from build123d import *

# Parameters (mm, degrees)
SKETCH_1_R          = 9.5
EXTRUDE_1_DEPTH     = 10
SKETCH_2_R          = 8.5
SKETCH_2_R_2        = 9.5
CUT_EXTRUDE_1_DEPTH = 5
SKETCH_3_R          = 3.25
SKETCH_3_R_2        = 2
EXTRUDE_2_DEPTH     = 5
SKETCH_4_W          = 16
SKETCH_4_H          = 2
CUT_EXTRUDE_2_DEPTH = 6
EXTRUDE_3_DEPTH     = 29.5
SKETCH_8_W          = 40
SKETCH_8_H          = 59
CUT_EXTRUDE_4_DEPTH = 8
SKETCH_9_R          = 9.5
CUT_EXTRUDE_5_DEPTH = 70
SKETCH_10_R         = 3.25
SKETCH_10_R_2       = 2
EXTRUDE_4_DEPTH     = 6


with BuildPart() as part:
    # Эскиз1 → Бобышка-Вытянуть1 (new body)
    with BuildSketch(Plane(origin=(0, 0, 0), x_dir=(1, 0, 0), z_dir=(0, 1, 0))):
        with BuildLine():
            Line((-20, 18), (20, 18))
            ThreePointArc((20, 18), (27.071067812, 15.071067812), (30, 8))
            Line((30, 8), (30, -2))
            ThreePointArc((30, -2), (27.071067812, -9.071067812), (20, -12))
            Line((20, -12), (-20, -12))
            ThreePointArc((-20, -12), (-27.071067812, -9.071067812), (-30, -2))
            Line((-30, -2), (-30, 8))
            ThreePointArc((-30, 8), (-27.071067812, 15.071067812), (-20, 18))
        make_face()
        with Locations(Location((-10, 0, 0), (0, 0, 270))):
            Circle(SKETCH_1_R, mode=Mode.SUBTRACT)
        with Locations(Location((10, 0, 0), (0, 0, 90))):
            Circle(SKETCH_1_R, mode=Mode.SUBTRACT)
    extrude_1 = extrude(amount=EXTRUDE_1_DEPTH)

    # Эскиз2 → Вырез-Вытянуть1 (cut)
    with BuildSketch(Plane(origin=(0, 10, 0), x_dir=(1, 0, 0), z_dir=(0, 1, 0))):
        with Locations((-20, -2)):
            Circle(SKETCH_2_R)
        with Locations((-20, 8)):
            Circle(SKETCH_2_R)
        with Locations(Location((-10, 0, 0), (0, 0, 270))):
            Circle(SKETCH_2_R_2)
        with BuildLine():
            Line((20, 16.5), (-20, 16.5))
            ThreePointArc((-20, 16.5), (-14.492370575, 14.474258113), (-11.609926002, 9.362592497))
            ThreePointArc((-11.609926002, 9.362592497), (-3.878084328, 7.26444413), (-0.5, 0))
            ThreePointArc((-0.5, 0), (-5.086783087, -8.13082404), (-14.417957802, -8.410210988))
            ThreePointArc((-14.417957802, -8.410210988), (-17.01979811, -9.960426917), (-20, -10.5))
            Line((-20, -10.5), (20, -10.5))
            ThreePointArc((20, -10.5), (17.01979811, -9.960426917), (14.417957802, -8.410210988))
            ThreePointArc((14.417957802, -8.410210988), (0.616398255, -1.48257151), (11.609926002, 9.362592497))
            ThreePointArc((11.609926002, 9.362592497), (14.492370575, 14.474258113), (20, 16.5))
        make_face()
        with Locations((-20, -2)):
            Circle(SKETCH_2_R)
        with Locations((-20, 8)):
            Circle(SKETCH_2_R)
        with Locations(Location((-10, 0, 0), (0, 0, 270))):
            Circle(SKETCH_2_R_2)
        with Locations((-20, -2)):
            Circle(SKETCH_2_R)
        with Locations((-20, 8)):
            Circle(SKETCH_2_R)
        with Locations(Location((-10, 0, 0), (0, 0, 270))):
            Circle(SKETCH_2_R_2)
        with BuildLine():
            ThreePointArc((-26.873863542, 3), (-28.08324935, 5.371106707), (-28.5, 8))
            Line((-28.5, 8), (-28.5, -2))
            ThreePointArc((-28.5, -2), (-28.08324935, 0.628893293), (-26.873863542, 3))
        make_face()
        with Locations((20, -2)):
            Circle(SKETCH_2_R)
        with Locations((20, 8)):
            Circle(SKETCH_2_R)
        with Locations(Location((10, 0, 0), (0, 0, 90))):
            Circle(SKETCH_2_R_2)
        with Locations((20, -2)):
            Circle(SKETCH_2_R)
        with Locations((20, 8)):
            Circle(SKETCH_2_R)
        with Locations(Location((10, 0, 0), (0, 0, 90))):
            Circle(SKETCH_2_R_2)
        with Locations((20, -2)):
            Circle(SKETCH_2_R)
        with Locations((20, 8)):
            Circle(SKETCH_2_R)
        with Locations(Location((10, 0, 0), (0, 0, 90))):
            Circle(SKETCH_2_R_2)
        with BuildLine():
            Line((28.5, -2), (28.5, 8))
            ThreePointArc((28.5, 8), (28.08324935, 5.371106707), (26.873863542, 3))
            ThreePointArc((26.873863542, 3), (28.08324935, 0.628893293), (28.5, -2))
        make_face()
    cut_extrude_1 = extrude(amount=-CUT_EXTRUDE_1_DEPTH, mode=Mode.SUBTRACT)

    # Эскиз3 → Бобышка-Вытянуть2 (add)
    with BuildSketch(Plane(origin=(0, 5, 0), x_dir=(1, 0, 0), z_dir=(0, 1, 0))):
        with Locations(Location((-23.5, 3, 0), (0, 0, 270))):
            Circle(SKETCH_3_R)
        with Locations(Location((-23.5, 3, 0), (0, 0, 270))):
            Circle(SKETCH_3_R_2, mode=Mode.SUBTRACT)
        with Locations(Location((23.5, 3, 0), (0, 0, 90))):
            Circle(SKETCH_3_R)
        with Locations(Location((23.5, 3, 0), (0, 0, 90))):
            Circle(SKETCH_3_R_2, mode=Mode.SUBTRACT)
    extrude_2 = extrude(amount=EXTRUDE_2_DEPTH)

    # Эскиз4 → Вырез-Вытянуть2 (cut, through all)
    with BuildSketch(Plane(origin=(0, 5, 0), x_dir=(1, 0, 0), z_dir=(0, 1, 0))):
        with Locations((0, 14)):
            Rectangle(SKETCH_4_W, SKETCH_4_H)
    cut_extrude_2 = extrude(amount=-CUT_EXTRUDE_2_DEPTH, mode=Mode.SUBTRACT)

    # Эскиз5 → Бобышка-Вытянуть3 (add)
    with BuildSketch(Plane.XZ):
        with BuildLine():
            Line((30, -8), (30, 2))
            ThreePointArc((30, 2), (27.071067812, 9.071067812), (20, 12))
            Line((20, 12), (-20, 12))
            ThreePointArc((-20, 12), (-27.071067812, 9.071067812), (-30, 2))
            Line((-30, 2), (-30, -8))
            ThreePointArc((-30, -8), (-27.071067812, -15.071067812), (-20, -18))
            Line((-20, -18), (20, -18))
            ThreePointArc((20, -18), (27.071067812, -15.071067812), (30, -8))
        make_face()
    extrude_3 = extrude(amount=EXTRUDE_3_DEPTH)

    # Зеркальное отражение5: Бобышка-Вытянуть1, Вырез-Вытянуть1, Бобышка-Вытянуть2, Вырез-Вытянуть2, Бобышка-Вытянуть3 across plane
    add(extrude_1.mirror(Plane(origin=(0, -29.5, 0), x_dir=(0, 0, 1), z_dir=(0, -1, 0))))
    add(cut_extrude_1.mirror(Plane(origin=(0, -29.5, 0), x_dir=(0, 0, 1), z_dir=(0, -1, 0))), mode=Mode.SUBTRACT)
    add(extrude_2.mirror(Plane(origin=(0, -29.5, 0), x_dir=(0, 0, 1), z_dir=(0, -1, 0))))
    add(cut_extrude_2.mirror(Plane(origin=(0, -29.5, 0), x_dir=(0, 0, 1), z_dir=(0, -1, 0))), mode=Mode.SUBTRACT)
    add(extrude_3.mirror(Plane(origin=(0, -29.5, 0), x_dir=(0, 0, 1), z_dir=(0, -1, 0))))

    # Эскиз8 → Вырез-Вытянуть4 (cut)
    with BuildSketch(Plane(origin=(0, 0, -18), x_dir=(-1, 0, 0), z_dir=(0, 0, -1))):
        with Locations((0, -29.5)):
            Rectangle(SKETCH_8_W, SKETCH_8_H)
    extrude(amount=-CUT_EXTRUDE_4_DEPTH, mode=Mode.SUBTRACT)

    # Эскиз9 → Вырез-Вытянуть5 (cut, through all)
    with BuildSketch(Plane(origin=(0, -59, 0), x_dir=(-1, 0, 0), z_dir=(0, -1, 0))):
        with Locations(Location((10, 0, 0), (0, 0, 270))):
            Circle(SKETCH_9_R)
        with Locations(Location((-10, 0, 0), (0, 0, 270))):
            Circle(SKETCH_9_R)
    extrude(amount=-CUT_EXTRUDE_5_DEPTH, mode=Mode.SUBTRACT)

    # Эскиз10 → Бобышка-Вытянуть4 (add)
    with BuildSketch(Plane(origin=(0, 0, -10), x_dir=(-1, 0, 0), z_dir=(0, 0, -1))):
        with Locations((-13.5, -52.5)):
            Circle(SKETCH_10_R)
        with Locations((-13.5, -52.5)):
            Circle(SKETCH_10_R_2, mode=Mode.SUBTRACT)
        with Locations(Location((13.5, -52.5, 0), (0, 0, 180))):
            Circle(SKETCH_10_R)
        with Locations(Location((13.5, -52.5, 0), (0, 0, 180))):
            Circle(SKETCH_10_R_2, mode=Mode.SUBTRACT)
        with Locations((13.5, -6.5)):
            Circle(SKETCH_10_R)
        with Locations((13.5, -6.5)):
            Circle(SKETCH_10_R_2, mode=Mode.SUBTRACT)
        with Locations(Location((-13.5, -6.5, 0), (0, 0, 180))):
            Circle(SKETCH_10_R)
        with Locations(Location((-13.5, -6.5, 0), (0, 0, 180))):
            Circle(SKETCH_10_R_2, mode=Mode.SUBTRACT)
    extrude(amount=EXTRUDE_4_DEPTH)


solid = part.part
Verification items for the finished model (mm, model axes). A direction names the side the tool comes from. Give positions to 0.01 mm unless a question says otherwise; leave off trailing zeros. Order: outer loops, then holes, each group sorted by start corner. A loop starts at its lowest first (then second) coordinate and runs counter-clockwise, first axis right, second up. Notation, with made-up numbers: M 38.5,46 L 66.5,46 A28 ccw 66.5,78 Z; hole C -25,58.5 d11. An arc over 180 degrees is marked long. Use one line per item in the form item = value. Start each with the question number.
Q1. Section check D-D (y = -11). Enter the section's corners in (x, z).
Q2. Scan lines: line 1 along X through (y, z) = (-61.05, 0); line 2 along Z through (x, y) = (9.5, -63.5); line 3 along Y through (x, z) = (13.5, -13.85). Record each from-to range of solid material in increasing order. Write a range as [from, to].
Q3. Section check B-B (x = 2.5). Enter the section's corners in (y, z).
Q4. Section check C-C (z = 4.75). Enter the section's corners in (x, y), then the cut area to 3 significant figures.
Q5. Access from +Z, -Z, +X, -X, +Y, -Y to the whole of each face (thin tool, end or side, straight path). Record for faces 4 (the flat face through (0, -64, -6)), 5 (the cylindrical face through (26.08, 7.54, -13.94)), 6 (the cylindrical face through (-14.205, -49.327, -12.958)), 7 (the flat face through (-26, -69, -3)), 8 (the flat face through (30, -30, -3)).
Q6. Mould release check, pull along Z, two halves, no side actions. Record for faces 1 (the flat face through (11, -52, -16)), 2 (the flat face through (0, -67, -16.5)), 3 (the cylindrical face through (14.205, -55.673, -12.958)): +Z half, -Z half, draft (parallel to the pull), parting line (faces both ways), or undercut.
Q7. Section check A-A (y = -52.5). Enter the section's corners in (x, z).
Q8. Go/stop test with flat-tipped pins: pin 1 Ø3 at (x, z) = (24.5, -2.5) entering from -Y; pin 2 Ø2 at (x, y) = (-3, -26.5) entering from -Z; pin 3 Ø17 at (x, z) = (-10, 0) entering from -Y; pin 4 Ø3 at (x, z) = (-23.5, -3) entering from -Y. Record where each tip stops, or that it passes through.
Evaluation:
q1.outline = M -30,-8 A10 ccw -20,-18 L -20,-10 L 20,-10 L 20,-18 A10 ccw 30,-8 L 30,2 A10 ccw 20,12 L -20,12 A10 ccw -30,2 Z; hole C -10,0 d19; hole C 10,0 d19
q2.line_1 = [-30, -19.5], [-0.5, 0.5], [19.5, 30]
q2.line_2 = [-18, -9.49], [9.49, 12]
q2.line_3 = [-64, -59], [-55.75, -54.5], [-50.5, -49.25], [-9.75, -8.5], [-4.5, -3.25], [0, 5]
q3.outline = M -69,-18 L -59,-18 L -59,-15 L -64,-15 L -64,-16.5 L -69,-16.5 Z; M -69,10.5 L -64,10.5 L -64,5.83 L 5,5.83 L 5,10.5 L 10,10.5 L 10,12 L -69,12 Z; M -64,-13 L -59,-13 L -59,-10 L 0,-10 L 0,-13 L 5,-13 L 5,-5.83 L -64,-5.83 Z; M 0,-18 L 10,-18 L 10,-16.5 L 5,-16.5 L 5,-15 L 0,-15 Z
q4.outline = M -29.61,-69 L -28.04,-69 L -28.04,-64 L -18.23,-64 L -18.23,5 L -28.04,5 L -28.04,10 L -29.61,10 Z; M -1.77,-64 L 1.77,-64 L 1.77,5 L -1.77,5 Z; M 18.23,-64 L 28.04,-64 L 28.04,-69 L 29.61,-69 L 29.61,10 L 28.04,10 L 28.04,5 L 18.23,5 Z
q4.area = 1,850 mm2
q5.face_4 = -Y
q5.face_5 = +Y
q5.face_6 = -Z
q5.face_7 = +Z, -Z, +X, -X, -Y
q5.face_8 = +Z, -Z, +X, +Y, -Y
q6.face_1 = -Z half
q6.face_2 = undercut
q6.face_3 = draft
q7.outline = M -30,-8 A10 ccw -20,-18 L -20,-10 L -16.75,-10 L -16.75,-16 L -15.5,-16 L -15.5,-10 L -11.5,-10 L -11.5,-16 L -10.25,-16 L -10.25,-10 L 10.25,-10 L 10.25,-16 L 11.5,-16 L 11.5,-10 L 15.5,-10 L 15.5,-16 L 16.75,-16 L 16.75,-10 L 20,-10 L 20,-18 A10 ccw 30,-8 L 30,2 A10 ccw 20,12 L -20,12 A10 ccw -30,2 Z; hole C -10,0 d19; hole C 10,0 d19
q8.pin_1 = -69
q8.pin_2 = -10
q8.pin_3 = through
q8.pin_4 = -64
